from build123d import *

# Parameters (mm, degrees)
ESBO_O1_W                         = 40
ESBO_O1_H                         = 20
RESSALTO_EXTRUS_O1_DEPTH          = 1
ESBO_O3_W                         = 40
ESBO_O3_H                         = 20
RESSALTO_EXTRUS_O2_DEPTH          = 2
CORTE_EXTRUS_O1_REACH             = 25.409
ESBO_O2_R                         = 2.5
ESBO_O2_R_2                       = 0.75
CORTE_EXTRUS_O1_DIRECTION_2_REACH = 25.409
ESBO_O4_W                         = 25
ESBO_O4_H                         = 35
ESBO_O4_R                         = 1.1
ESBO_O4_W_2                       = 13
ESBO_O4_H_2                       = 23
ESBO_O4_H_3                       = 3
RESSALTO_EXTRUS_O3_DEPTH          = 3
FILLET2_R                         = 3


with BuildPart() as part:
    # Esbo_o1 → Ressalto-extrus_o1 (new body)
    with BuildSketch(Plane.XY):
        with Locations((0, -2)):
            Rectangle(ESBO_O1_W, ESBO_O1_H)
    extrude(amount=-RESSALTO_EXTRUS_O1_DEPTH)

    # Esbo_o3 → Ressalto-extrus_o2 (add)
    with BuildSketch(Plane.XY):
        with Locations((0, -2)):
            Rectangle(ESBO_O3_W, ESBO_O3_H)
    extrude(amount=RESSALTO_EXTRUS_O2_DEPTH)

    # Corte-extrus_o1: up to this face of the body (flat: up to its plane)
    corte_extrus_o1_end = Plane(part.part.faces().sort_by_distance((0, -2, 2))[0])
    # Esbo_o2 → Corte-extrus_o1 (cut, up to the picked face)
    with BuildSketch(Plane.XY, mode=Mode.PRIVATE) as corte_extrus_o1_sk1:
        with Locations(Location((0, -5, 0), (0, 0, 180))):
            Circle(ESBO_O2_R)
    corte_extrus_o1_tool1 = split(extrude(corte_extrus_o1_sk1.sketch, amount=CORTE_EXTRUS_O1_REACH, mode=Mode.PRIVATE), bisect_by=corte_extrus_o1_end, keep=Keep.BOTH, mode=Mode.PRIVATE)
    # Esbo_o2 → Corte-extrus_o1 (cut, up to the picked face)
    with BuildSketch(Plane.XY, mode=Mode.PRIVATE) as corte_extrus_o1_sk2:
        with Locations(Location((-8.5, -5, 0), (0, 0, 180))):
            Circle(ESBO_O2_R_2)
    corte_extrus_o1_tool2 = split(extrude(corte_extrus_o1_sk2.sketch, amount=CORTE_EXTRUS_O1_REACH, mode=Mode.PRIVATE), bisect_by=corte_extrus_o1_end, keep=Keep.BOTH, mode=Mode.PRIVATE)
    corte_extrus_o1_1 = corte_extrus_o1_tool1.solids().sort_by(Axis((0, -5, 0), (0, 0, 1)))[0]
    add(corte_extrus_o1_1, mode=Mode.SUBTRACT)
    corte_extrus_o1_2 = corte_extrus_o1_tool2.solids().sort_by(Axis((-8.5, -5, 0), (0, 0, 1)))[0]
    add(corte_extrus_o1_2, mode=Mode.SUBTRACT)
    corte_extrus_o1 = corte_extrus_o1_1 + corte_extrus_o1_2  # Corte-extrus_o1 as one shape, for the pattern or mirror that repeats it

    # Corte-extrus_o1 direction 2: up to this face of the body (flat: up to its plane)
    corte_extrus_o1_direction_2_end = Plane(part.part.faces().sort_by_distance((0, -2, -1))[0])
    # Esbo_o2 → Corte-extrus_o1 direction 2 (cut, up to the picked face)
    with BuildSketch(Plane.XY, mode=Mode.PRIVATE) as corte_extrus_o1_direction_2_sk1:
        with Locations(Location((0, -5, 0), (0, 0, 180))):
            Circle(ESBO_O2_R)
    corte_extrus_o1_direction_2_tool1 = split(extrude(corte_extrus_o1_direction_2_sk1.sketch, amount=-CORTE_EXTRUS_O1_DIRECTION_2_REACH, mode=Mode.PRIVATE), bisect_by=corte_extrus_o1_direction_2_end, keep=Keep.BOTH, mode=Mode.PRIVATE)
    # Esbo_o2 → Corte-extrus_o1 direction 2 (cut, up to the picked face)
    with BuildSketch(Plane.XY, mode=Mode.PRIVATE) as corte_extrus_o1_direction_2_sk2:
        with Locations(Location((-8.5, -5, 0), (0, 0, 180))):
            Circle(ESBO_O2_R_2)
    corte_extrus_o1_direction_2_tool2 = split(extrude(corte_extrus_o1_direction_2_sk2.sketch, amount=-CORTE_EXTRUS_O1_DIRECTION_2_REACH, mode=Mode.PRIVATE), bisect_by=corte_extrus_o1_direction_2_end, keep=Keep.BOTH, mode=Mode.PRIVATE)
    corte_extrus_o1_direction_2_1 = corte_extrus_o1_direction_2_tool1.solids().sort_by(Axis((0, -5, 0), (0, 0, -1)))[0]
    add(corte_extrus_o1_direction_2_1, mode=Mode.SUBTRACT)
    corte_extrus_o1_direction_2_2 = corte_extrus_o1_direction_2_tool2.solids().sort_by(Axis((-8.5, -5, 0), (0, 0, -1)))[0]
    add(corte_extrus_o1_direction_2_2, mode=Mode.SUBTRACT)
    corte_extrus_o1_direction_2 = corte_extrus_o1_direction_2_1 + corte_extrus_o1_direction_2_2  # Corte-extrus_o1 direction 2 as one shape, for the pattern or mirror that repeats it

    # Esbo_o4 → Ressalto-extrus_o3 (add)
    # profile 1 of 2: a face of its own
    with BuildSketch(Plane(origin=(0, 8, 0), x_dir=(1, 0, 0), z_dir=(0, 1, 0))):
        with Locations((0, -19.5)):
            Rectangle(ESBO_O4_W, ESBO_O4_H)
        with Locations(Location((0, -33.25, 0), (0, 0, 180))):
            Circle(ESBO_O4_R, mode=Mode.SUBTRACT)
        with Locations((0, -20)):
            Rectangle(ESBO_O4_W_2, ESBO_O4_H_2, mode=Mode.SUBTRACT)
        with Locations(Location((0, -6.75, 0), (0, 0, 180))):
            Circle(ESBO_O4_R, mode=Mode.SUBTRACT)
    # profile 2 of 2: a face of its own
    with BuildSketch(Plane(origin=(0, 8, 0), x_dir=(1, 0, 0), z_dir=(0, 1, 0))):
        with Locations((0, -0.5)):
            Rectangle(ESBO_O4_W, ESBO_O4_H_3)
    extrude(amount=-RESSALTO_EXTRUS_O3_DEPTH)

    # Mirror1: Corte-extrus_o1, Corte-extrus_o1 direction 2 across plane
    add(corte_extrus_o1.mirror(Plane(origin=(0, 0, 0), x_dir=(0, 0, 1), z_dir=(1, 0, 0))), mode=Mode.SUBTRACT)
    add(corte_extrus_o1_direction_2.mirror(Plane(origin=(0, 0, 0), x_dir=(0, 0, 1), z_dir=(1, 0, 0))), mode=Mode.SUBTRACT)

    # Fillet2
    fillet2_edges = [part.edges().sort_by_distance(p)[0] for p in [
        (0, 8, -1),
        (0, 5, 2),
        (12.5, 6.5, 2),
        (-12.5, 6.5, 2),
        (-12.5, 6.5, 37),
        (12.5, 6.5, 37),
        (-20, -12, 0.5),
        (-20, 8, 0.5),
        (20, 8, 0.5),
        (20, -12, 0.5),
    ]]
    fillet(fillet2_edges, radius=FILLET2_R - 0.0001)  # a hair under: the kernel refuses the full size


solid = part.part
Geometry: final body of the model. Coordinates: model frame, mm. A direction names the side the tool comes from. Give positions to 0.01 mm unless a question says otherwise; leave off trailing zeros. Write each loop counter-clockwise with the first axis right and the second up, starting at its lowest first coordinate (ties: lowest second). Pieces come first, ordered by that corner, then holes. Notation, with made-up numbers: (68.25, -25) -> (74.25, -25) arc R6 ccw to (74.25, -17) -> close; hole circle Ø4 at (-9.75, -33). An arc over 180 degrees is marked (long way). Answer as a JSON object with one key per item and string values.
1. Mould query, pull axis Z, two halves, no side actions, for faces 4 (the flat face through (0, -2, 2)), 5 (the cylindrical face through (-0.59, 6.52, 7.68)), 6 (the flat face through (-8, 8, 19)). Classes: pulls with the +Z half, pulls with the -Z half, needs draft (parallel to the pull), parting line crosses it, or undercut.
Ans:
{"face 4": "pulls with the +Z half", "face 5": "undercut", "face 6": "needs draft"}
2. Cut plane A-A on z = 12. Output: boundary loops of the cut face in (x, y), and give its area (3 significant figures).
Ans:
{"outline": "(-12.5, 5) -> (-6.5, 5) -> (-6.5, 8) -> (-12.5, 8) -> close; (6.5, 5) -> (12.5, 5) -> (12.5, 8) -> (6.5, 8) -> close", "area": "36.0 mm^2"}
3. Access query for faces 1 (the flat face through (-6.5, 7, 20)), 2 (the flat face through (-12.5, 7, 20)), 3 (the cylindrical face through (11.6, 6.48, 36.14)). Directions: +Z, -Z, +X, -X, +Y, -Y. A direction counts if a zero-diameter tool reaches every point of the face in a straight line with its end or side. Return the directions, or none.
Ans:
{"face 1": "+Y, -Y", "face 2": "+Z, -X, +Y, -Y", "face 3": "+Z, +X, +Y, -Y"}
4. Cut plane C-C on x = 4. Output: boundary loops of the cut face in (y, z).
Ans:
{"outline": "(-12, -1) -> (5, -1) arc R3 ccw to (8, 2) -> (8, 8.5) -> (5, 8.5) -> (5, 5) arc R3 cw to (2, 2) -> (-12, 2) -> close; (5, 31.5) -> (8, 31.5) -> (8, 37) -> (5, 37) -> close"}
5. Contact query for flat-ended pins moving along their axis: pin 1 (6 mm diameter, centred on y = 4.5, z = 13, fed in from -X); pin 2 (0.9 mm diameter, centred on x = -8.5, y = -5, fed in from +Z); pin 3 (1.7 mm diameter, centred on x = -8.5, y = -5, fed in from +Z); pin 4 (1.5 mm diameter, centred on y = 7, z = 24.5, fed in from +X). Output: stop coordinate, or through.
Ans:
{"pin 1": "stops at x = -12.5", "pin 2": "passes through", "pin 3": "stops at z = 2", "pin 4": "stops at x = 12.5"}
6. Cut plane D-D on y = 6.25. Output: boundary loops of the cut face in (x, z), and give its area (3 significant figures).
Ans:
{"outline": "(-19.73, -0.73) -> (19.73, -0.73) -> (19.73, 2) -> (15.5, 2) arc R3 cw to (12.5, 5) -> (12.5, 34) arc R3 ccw to (9.5, 37) -> (-9.5, 37) arc R3 ccw to (-12.5, 34) -> (-12.5, 5) arc R3 cw to (-15.5, 2) -> (-19.73, 2) -> close; hole (-6.5, 8.5) -> (6.5, 8.5) -> (6.5, 31.5) -> (-6.5, 31.5) -> close; hole circle Ø2.2 at (0, 6.75); hole circle Ø2.2 at (0, 33.25)", "area": "676 mm^2"}
7. Ray query, probe 1 along Z at (x, y) = (0, 6.95); probe 2 along Z at (x, y) = (9.5, 1.75); probe 3 along X at (y, z) = (5.5, 18). Return the intervals inside material, ascending. Write a range as from..to.
Ans:
{"probe 1": "z = -0.28..5.65, 7.85..8.5, 31.5..32.15, 34.35..37", "probe 2": "z = -1..2", "probe 3": "x = -12.5..-6.5, 6.5..12.5"}
8. Cut plane B-B on x = 0. Output: boundary loops of the cut face in (y, z), and give its area (3 significant figures).
Ans:
{"outline": "(-12, -1) -> (-7.5, -1) -> (-7.5, 2) -> (-12, 2) -> close; (-2.5, -1) -> (5, -1) arc R3 ccw to (8, 2) -> (8, 5.65) -> (5, 5.65) -> (5, 5) arc R3 cw to (2, 2) -> (-2.5, 2) -> close; (5, 7.85) -> (8, 7.85) -> (8, 8.5) -> (5, 8.5) -> close; (5, 31.5) -> (8, 31.5) -> (8, 32.15) -> (5, 32.15) -> close; (5, 34.35) -> (8, 34.35) -> (8, 37) -> (5, 37) -> close", "area": "67.8 mm^2"}
